Verification items for the finished model (mm, model axes). A direction names the side the tool comes from. Round coordinates to 2 decimals unless told otherwise and drop trailing zeros. Loops run counter-clockwise (first coordinate to the right, second up) from the corner with the lowest first, then second, coordinate; pieces in that order, holes last. Notation, with made-up numbers: (-25, 53) -> (11, 53) arc R14 ccw to (11, 71) -> close; hole circle Ø10 at (85.25, -4.5). An arc over 180 degrees is marked (long way). Write item = value, one per line. Start each with the question number.
```python
from build123d import *

# Parameters (mm, degrees)
F2_R     = 4.826
F3_DEPTH = 38.1
F2_R_2   = 11.176
F4_DEPTH = 6.35


with BuildPart() as f1:
    # F0 (on Front) → F1 (revolve)
    with BuildSketch(Plane.XZ):
        Polygon((-16.98684, -24.258915), (-10.63684, -24.258915), (-10.63684, -17.908915), (0.589637, 13.841085), (-1.11184, 20.191085), (-16.98684, 20.191085), align=None)
    revolve(axis=Axis((-16.98684, 0, -2.033915), (0, 0, -1)))

    # F2 (on face) → F3 (cut)
    with BuildSketch(Plane.XY.offset(20.191085)):
        with Locations((-16.900598, 0)):
            Circle(F2_R)
    extrude(amount=-F3_DEPTH, mode=Mode.SUBTRACT)

    # F2 (on face) → F4 (cut)
    with BuildSketch(Plane.XY.offset(20.191085)):
        with Locations((-16.900598, 0)):
            Circle(F2_R_2)
        with Locations((-16.900598, 0)):
            Circle(F2_R, mode=Mode.SUBTRACT)
    extrude(amount=-F4_DEPTH, mode=Mode.SUBTRACT)


solid = f1.part
```
(1) Depth check by flat-ended pin: pin 1 Ø10 at (y, z) = (0, -5) entering from +X; pin 2 Ø10 at (x, y) = (-10.5, 2.5) entering from -Z; pin 3 Ø3 at (x, y) = (-19, -0.5) entering from +Z; pin 4 Ø12 at (x, z) = (-6, -13) entering from -Y. Enter the tip coordinate at first touch or a pass-through.
(2) Access from +Z, -Z, +X, -X, +Y, -Y to the whole of each face (thin tool, end or side, straight path). Record for faces 5 (the flat face through (-17, 0, -24.259)), 6 (the cylindrical face through (-21.67, -4.29, -21.04)), 7 (the flat face through (-12, -2, 13.841)).
(3) Section check A-A on y = 0. Enter the section's corners in (x, z), then the cut area to 3 significant figures.
(4) Draft check along Y on faces 1 (the conical face through (-25.55, 6.57, -5.34)), 2 (the flat face through (-14, -11, 20.191)), 3 (the flat face through (-17, 0, -17.909)), 4 (the cylindrical face through (-21.722, 0.212, -1.812)). Enter one of: +Y half, -Y half, draft (parallel to the pull), parting line (faces both ways), or undercut.
(5) Section check C-C on z = -19.5. Enter the section's corners in (x, y), then the cut area to 3 significant figures.
(6) Scan lines: line 1 (Z direction, x = -17.5, y = -6); line 2 (Y direction, x = -7.5, z = 17.5); line 3 (Y direction, x = -20.5, z = 12.5). Record each from-to range of solid material in increasing order. Write a range as [from, to].
(7) Section check D-D on z = 6. Enter the section's corners in (x, y).
(8) Section check B-B on z = -3. Enter the section's corners in (x, y).
Computed values:
q1.pin_1 = -4.3
q1.pin_2 = -24.26
q1.pin_3 = -17.91
q1.pin_4 = -7.08
q2.face_5 = -Z, +X, -X, +Y, -Y
q2.face_6 = -Z
q2.face_7 = +Z
q3.outline = (-34.56, 13.84) -> (-23.34, -17.91) -> (-23.34, -24.26) -> (-10.64, -24.26) -> (-10.64, -17.91) -> (0.59, 13.84) -> (-1.11, 20.19) -> (-5.72, 20.19) -> (-5.72, 13.84) -> (-12.07, 13.84) -> (-12.07, -17.91) -> (-21.73, -17.91) -> (-21.73, 13.84) -> (-28.08, 13.84) -> (-28.08, 20.19) -> (-32.86, 20.19) -> close
q3.area = 604 mm²
q4.face_1 = parting line
q4.face_2 = draft
q4.face_3 = undercut
q4.face_4 = undercut
q5.outline = circle Ø12.7 at (-16.99, 0)
q5.area = 127 mm²
q6.line_1 = [-24.26, 13.84]
q6.line_2 = [-13.62, -6.04], [6.04, 13.62]
q6.line_3 = [-16.74, -3.21], [3.21, 16.74]
q7.outline = circle Ø29.61 at (-16.99, 0); hole circle Ø9.65 at (-16.9, 0)
q8.outline = circle Ø23.24 at (-16.99, 0); hole circle Ø9.65 at (-16.9, 0)
